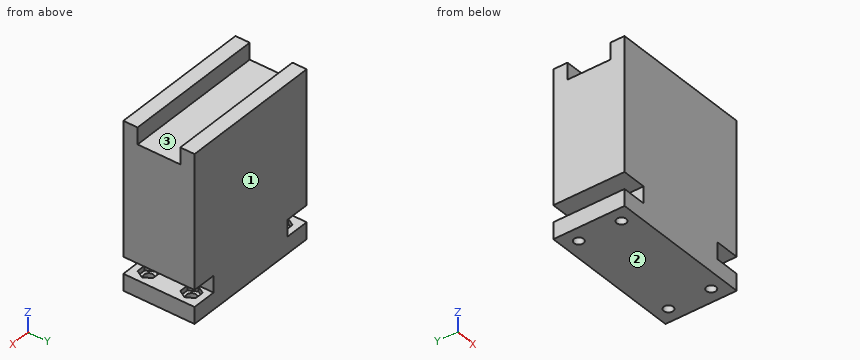
from build123d import *

# Parameters (mm, degrees)
F0_W     = 60.1
F0_H     = 30
F0_R     = 2
F1_DEPTH = 5
F2_W     = 60.1
F2_H     = 30
F3_DEPTH = 2
F4_W     = 39.7
F4_H     = 30
F5_DEPTH = 7
F6_W     = 60.1
F6_H     = 30
F7_DEPTH = 49
F8_W     = 60.1
F8_H     = 6
F9_DEPTH = 7


with BuildPart() as f1:
    # F0 (on Top) → F1 (new body)
    with BuildSketch(Plane.XY):
        Rectangle(F0_W, F0_H)
        with Locations((-24.05, -9)):
            Circle(F0_R, mode=Mode.SUBTRACT)
        with Locations((24.05, -9)):
            Circle(F0_R, mode=Mode.SUBTRACT)
        with Locations((-24.05, 9)):
            Circle(F0_R, mode=Mode.SUBTRACT)
        with Locations((24.05, 9)):
            Circle(F0_R, mode=Mode.SUBTRACT)
    extrude(amount=F1_DEPTH)

    # F2 (on face) → F3 (join)
    with BuildSketch(Plane.XY.offset(5)):
        Rectangle(F2_W, F2_H)
        Polygon((-25.9263883749, -5.75), (-22.1736116251, -5.75), (-20.2972232503, -9), (-22.1736116251, -12.25), (-25.9263883749, -12.25), (-27.8027767497, -9), align=None, mode=Mode.SUBTRACT)
        Polygon((20.2972232503, -9), (22.1736116251, -5.75), (25.9263883749, -5.75), (27.8027767497, -9), (25.9263883749, -12.25), (22.1736116251, -12.25), align=None, mode=Mode.SUBTRACT)
        Polygon((-22.1736116251, 5.75), (-25.9263883749, 5.75), (-27.8027767497, 9), (-25.9263883749, 12.25), (-22.1736116251, 12.25), (-20.2972232503, 9), align=None, mode=Mode.SUBTRACT)
        Polygon((25.9263883749, 5.75), (22.1736116251, 5.75), (20.2972232503, 9), (22.1736116251, 12.25), (25.9263883749, 12.25), (27.8027767497, 9), align=None, mode=Mode.SUBTRACT)
    extrude(amount=F3_DEPTH)

    # F4 (on face) → F5 (join)
    with BuildSketch(Plane.XY.offset(7)):
        Rectangle(F4_W, F4_H)
    extrude(amount=F5_DEPTH)

    # F6 (on face) → F7 (join)
    with BuildSketch(Plane.XY.offset(14)):
        Rectangle(F6_W, F6_H)
    extrude(amount=F7_DEPTH)

    # F8 (on face) → F9 (join)
    with BuildSketch(Plane.XY.offset(63)):
        with Locations((0, 12)):
            Rectangle(F8_W, F8_H)
        with Locations((0, -12)):
            Rectangle(F8_W, F8_H)
    extrude(amount=F9_DEPTH)


solid = f1.part
Verification items for the finished model (mm, model axes). Face numbers are marked on the shaded views. Round coordinates to 2 decimals unless told otherwise and drop trailing zeros. Loops run counter-clockwise (first coordinate to the right, second up) from the corner with the lowest first, then second, coordinate; pieces in that order, holes last. Notation, with made-up numbers: (8.5, -19.5) - (37.5, -19.5) arc R26 ccw to (37.5, 15.5) - close; hole circle Ø6 at (-38, -35.5). An arc over 180 degrees is marked (long way). Answer in a Markdown table with one row per item. Add a question column.
Q1. Material ranges on line 1 (Y direction, x = -24.05, z = 3.15); line 2 (Z direction, x = 3.5, y = -4); line 3 (X direction, y = 9, z = 10.5), recorded low to high.
Q2. Gauge pin test, flat end, axial feed: pin 1 (5 mm diameter, centred on x = -23.5, y = 0, fed in from +Z). Record the tip position at first contact, or that the pin passes through.
Q3. Section check A-A on x = -24.05. Enter the section's corners in (y, z), plus the area to 3 significant figures.
Q4. Release check for a two-part mould opening along Y. For the marked faces 1, 2 and 3 record: pulls with the +Y half, pulls with the -Y half, needs draft (parallel to the pull), parting line crosses it, or undercut.
Q5. Section check B-B on y = 1.75. Enter the section's corners in (x, z), plus the area to 3 significant figures.
Found:
| question | item | result |
|---|---|---|
| 1 | line 1 | y = -15 to -11, -7 to 7, 11 to 15 |
| 1 | line 2 | z = 0 to 63 |
| 1 | line 3 | x = -19.85 to 19.85 |
| 2 | pin 1 | stops at z = 63 |
| 3 | outline | (-15, 0) - (-11, 0) - (-11, 5) - (-12.25, 5) - (-12.25, 7) - (-15, 7) - close; (-15, 14) - (15, 14) - (15, 70) - (9, 70) - (9, 63) - (-9, 63) - (-9, 70) - (-15, 70) - close; (-7, 0) - (7, 0) - (7, 5) - (5.75, 5) - (5.75, 7) - (-5.75, 7) - (-5.75, 5) - (-7, 5) - close; (11, 0) - (15, 0) - (15, 7) - (12.25, 7) - (12.25, 5) - (11, 5) - close |
| 3 | area | 1,700 mm² |
| 4 | face 1 | pulls with the +Y half |
| 4 | face 2 | needs draft |
| 4 | face 3 | undercut |
| 5 | outline | (-30.05, 0) - (30.05, 0) - (30.05, 7) - (19.85, 7) - (19.85, 14) - (30.05, 14) - (30.05, 63) - (-30.05, 63) - (-30.05, 14) - (-19.85, 14) - (-19.85, 7) - (-30.05, 7) - close |
| 5 | area | 3,640 mm² |
